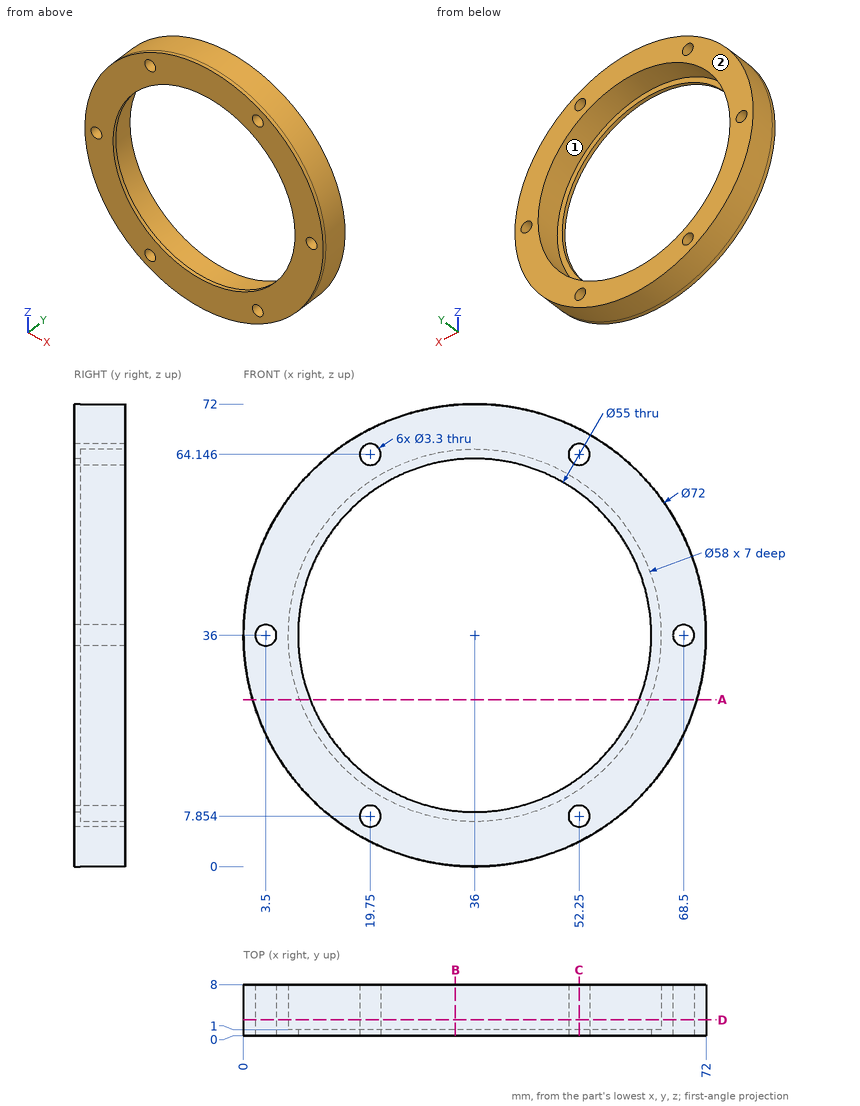
Verification items for this drawing (mm, ordinates from the low corner). Coordinates: 2 decimals unless noted, no trailing zeros. Loops run counter-clockwise (first coordinate to the right, second up) from the corner with the lowest first, then second, coordinate; pieces in that order, holes last. Notation, with made-up numbers: (85.25, 27) - (137.25, 27) arc R26 cw to (137.25, 45) - close; hole circle Ø8 at (22.5, -22). An arc over 180 degrees is marked (long way). Use one line per item in the form item = value. Start each with the question number.
Item 1: Section check B-B, the plane x = 33. Enter the section's corners in (y, z) (1 decimal), and give its area (4 significant figures).
Item 2: Mould release check, pull along X, two halves, no side actions. Record for the marked faces 1 and 2: +X half, -X half, draft (parallel to the pull), parting line (faces both ways), or undercut.
Item 3: Gauge pin test, flat ends, axial feed: pin 1 (1.5 mm diameter, centred on y = 5.5, z = 48, fed in from +X); pin 2 (4 mm diameter, centred on y = 6.5, z = 37.5, fed in from +X). Record the tip position at first contact, or that the pin passes through.
Item 4: Thickness scan on probe 1 along X at (y, z) = (2, 36); probe 2 along Z at (x, y) = (19.75, 5.75); probe 3 along Z at (x, y) = (21, 1.5) (1 decimal). Record the ranges inside material, lowest first.
Item 5: Section check D-D, the plane y = 2.5. Enter the section's corners in (x, z), and give its area (3 significant figures).
Item 6: Section check C-C, the plane x = 52.25. Enter the section's corners in (y, z) (1 decimal).
Item 7: Section check A-A, the plane z = 26. Enter the section's corners in (x, y), and give its area (3 significant figures).
Computed:
q1.outline = (0, 0.1) - (8, 0.1) - (8, 7.2) - (1, 7.2) - (1, 8.7) - (0, 8.7) - close; (0, 63.3) - (1, 63.3) - (1, 64.8) - (8, 64.8) - (8, 71.9) - (0, 71.9) - close
q1.area = 115.5 mm2
q2.face_1 = undercut
q2.face_2 = draft
q3.pin_1 = 70.2
q3.pin_2 = 72
q4.probe_1 = 0 to 1.85, 5.15 to 7, 65 to 66.85, 70.15 to 72
q4.probe_2 = 3.88 to 6.2, 9.5 to 11.98, 60.02 to 62.5, 65.8 to 68.12
q4.probe_3 = 3.3 to 6.8, 8.9 to 11.2, 60.8 to 63.1, 65.2 to 68.7
q5.outline = circle Ø72 at (36, 36); hole circle Ø3.3 at (3.5, 36); hole circle Ø58 at (36, 36); hole circle Ø3.3 at (19.75, 7.85); hole circle Ø3.3 at (19.75, 64.15); hole circle Ø3.3 at (52.25, 7.85); hole circle Ø3.3 at (52.25, 64.15); hole circle Ø3.3 at (68.5, 36)
q5.area = 1,380 mm2
q6.outline = (0, 3.9) - (8, 3.9) - (8, 6.2) - (0, 6.2) - close; (0, 9.5) - (8, 9.5) - (8, 12) - (1, 12) - (1, 13.8) - (0, 13.8) - close; (0, 58.2) - (1, 58.2) - (1, 60) - (8, 60) - (8, 62.5) - (0, 62.5) - close; (0, 65.8) - (8, 65.8) - (8, 68.1) - (0, 68.1) - close
q7.outline = (1.42, 0) - (10.38, 0) - (10.38, 1) - (8.78, 1) - (8.78, 8) - (1.42, 8) - close; (61.62, 0) - (70.58, 0) - (70.58, 8) - (63.22, 8) - (63.22, 1) - (61.62, 1) - close
q7.area = 121 mm2
